from build123d import *

# Parameters (mm, degrees)
F0_W     = 30
F0_H     = 10
F1_DEPTH = 60
F2_W     = 108
F2_H     = 39.921402
F3_DEPTH = 150
F4_W     = 25.141022
F4_H     = 108
F5_DEPTH = 6


with BuildPart() as f1:
    # F0 (on Front) → F1 (new body, symmetric)
    with BuildSketch(Plane.XZ):
        Polygon((-15, 5), (15, 5), (7.140478, 25), (4, 25), (4, 10), (-4, 10), (-4, 25), (-7.140478, 25), align=None)
        Rectangle(F0_W, F0_H)
    extrude(amount=F1_DEPTH, both=True)

    # F2 (on Right) → F3 (cut, symmetric)
    with BuildSketch(Plane.YZ):
        with Locations((0, 24.950191)):
            Rectangle(F2_W, F2_H)
    extrude(amount=F3_DEPTH, both=True, mode=Mode.SUBTRACT)

    # F4 (on face) → F5 (cut)
    with BuildSketch(Plane.XY.offset(4.98949)):
        Rectangle(F4_W, F4_H)
    extrude(amount=-F5_DEPTH, mode=Mode.SUBTRACT)


solid = f1.part
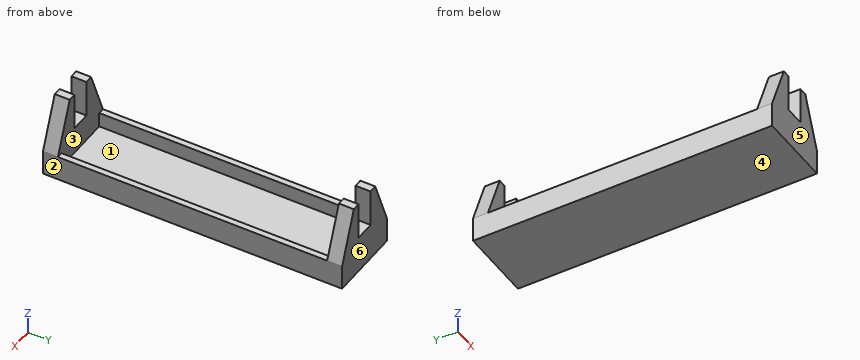
Geometry: final body of the model. Coordinates: model frame, mm. Face numbers are marked on the shaded views. A direction names the side the tool comes from. Give positions to 0.01 mm unless a question says otherwise; leave off trailing zeros. Loops run counter-clockwise (first coordinate to the right, second up) from the corner with the lowest first, then second, coordinate; pieces in that order, holes last. Notation, with made-up numbers: M -28,30 L -2,30 A6 ccw -2,41 Z; hole C -4.5,-27.5 d6. An arc over 180 degrees is marked long. Put each result on its own line as item: value. Start each with the question number.
1) Contact query for flat-ended pins moving along their axis: pin 1 (4 mm diameter, centred on x = -9, y = -48, fed in from +Z); pin 2 (1.8 mm diameter, centred on y = 56, z = 21, fed in from -X); pin 3 (3 mm diameter, centred on y = -57, z = 19, fed in from -X); pin 4 (6.5 mm diameter, centred on x = -1.5, y = 55.5, fed in from +Z). Output: stop coordinate, or through.
2) Ray query, line 1 along Y through (x, z) = (11, 0.5); line 2 along X through (y, z) = (-4, 0.5); line 3 along Z through (x, y) = (1, 16). Return the intervals inside material, ascending.
3) Cut plane C-C (z = 6.5). Output: boundary loops of the cut face in (x, y).
4) Cut plane D-D (x = 9.5). Output: boundary loops of the cut face in (y, z).
5) Cut plane A-A (z = 16). Output: boundary loops of the cut face in (x, y), then the cut area to 3 significant figures.
6) Cut plane B-B (y = -35). Output: boundary loops of the cut face in (x, z), then the cut area to 3 significant figures.
7) Access query for the marked faces 1 and 2. Directions: +Z, -Z, +X, -X, +Y, -Y. A direction counts if a zero-diameter tool reaches every point of the face in a straight line with its end or side. Return the directions, or none.
8) Pull-direction query (Y, two-part tool) for the marked faces 3, 4, 5 and 6; classes: pulls with the +Y half, pulls with the -Y half, needs draft (parallel to the pull), parting line crosses it, or undercut.
Verdict:
1. pin 1: z = -1.01
1. pin 2: x = -9.07
1. pin 3: x = -10.09
1. pin 4: z = 25
2. line 1: -60 to -54, 54 to 60
2. line 2: -15 to -12.57, 12.57 to 15
2. line 3: -5 to -1.01
3. outline: M -14.41,-60 L 14.41,-60 L 14.41,-54 L -14.41,-54 Z; M -14.41,54 L 14.41,54 L 14.41,60 L -14.41,60 Z
4. outline: M -60,-5 L 60,-5 L 60,19 L 54,19 L 54,-1.01 L -54,-1.01 L -54,19 L -60,19 Z
5. outline: M -10.68,-60 L -4,-60 L -4,-54 L -10.68,-54 Z; M -10.68,54 L -4,54 L -4,60 L -10.68,60 Z; M 4,-60 L 10.68,-60 L 10.68,-54 L 4,-54 Z; M 4,54 L 10.68,54 L 10.68,60 L 4,60 Z
5. area: 160 mm2
6. outline: M -15,-5 L 15,-5 L 15,4.99 L 12.57,4.99 L 12.57,-1.01 L -12.57,-1.01 L -12.57,4.99 L -15,4.99 Z
6. area: 149 mm2
7. face 1: +Z
7. face 2: +Z, -Z, +X, +Y, -Y
8. face 3: undercut
8. face 4: needs draft
8. face 5: pulls with the -Y half
8. face 6: pulls with the +Y half
